from build123d import *

# Parameters (mm, degrees)
EXTRUDE_1_DEPTH     = 5
EXTRUDE_2_DEPTH     = 7
SKETCH_3_R          = 1.5
CUT_EXTRUDE_1_DEPTH = 10
SKETCH_4_R          = 1.6
CUT_EXTRUDE_2_DEPTH = 3.5
SKETCH_5_W          = 8
SKETCH_5_H          = 4
CUT_EXTRUDE_4_DEPTH = 21.784609691
FILLET_1_R          = 5


with BuildPart() as part:
    # 草图1 → 凸台-拉伸1 (new body)
    with BuildSketch(Plane(origin=(0, 0, 0), x_dir=(1, 0, 0), z_dir=(0, 1, 0))):
        with BuildLine():
            ThreePointArc((12, 0), (0, 12), (-12, 0))
            Line((-12, 0), (12, 0))
        make_face()
        with BuildLine():
            ThreePointArc((-12, 0), (-11.422817781, -3.676851089), (-9.746794345, -7))
            Line((-9.746794345, -7), (9.746794345, -7))
            ThreePointArc((9.746794345, -7), (11.422817781, -3.676851089), (12, 0))
            Line((12, 0), (-12, 0))
        make_face()
        with BuildLine():
            Line((-12, 0), (-12, -7))
            Line((-12, -7), (-9.746794345, -7))
            ThreePointArc((-9.746794345, -7), (-11.422817781, -3.676851089), (-12, 0))
        make_face()
        with BuildLine():
            Line((9.746794345, -7), (-9.746794345, -7))
            ThreePointArc((-9.746794345, -7), (0, -12), (9.746794345, -7))
        make_face()
        with BuildLine():
            ThreePointArc((12, 0), (11.422817781, -3.676851089), (9.746794345, -7))
            Line((9.746794345, -7), (12, -7))
            Line((12, -7), (12, 0))
        make_face()
    extrude(amount=EXTRUDE_1_DEPTH)

    # 草图2 → 凸台-拉伸2 (add)
    with BuildSketch(Plane(origin=(0, 5, 0), x_dir=(1, 0, 0), z_dir=(0, 1, 0))):
        with BuildLine():
            Line((-12, 0), (-12, -7))
            Line((-12, -7), (-9.746794345, -7))
            Line((-9.746794345, -7), (9.746794345, -7))
            Line((9.746794345, -7), (12, -7))
            Line((12, -7), (12, 0))
            ThreePointArc((12, 0), (11.827182716, 2.029223745), (11.313708499, 4))
            Line((11.313708499, 4), (-11.313708499, 4))
            ThreePointArc((-11.313708499, 4), (-11.827182716, 2.029223745), (-12, 0))
        make_face()
    extrude(amount=EXTRUDE_2_DEPTH)

    # 草图3 → 切除-拉伸1 (cut)
    with BuildSketch(Plane.XZ):
        with Locations(Location((9, 0, 0), (0, 0, 270))):
            Circle(SKETCH_3_R)
        with Locations(Location((-9, 0, 0), (0, 0, 90))):
            Circle(SKETCH_3_R)
    extrude(amount=-CUT_EXTRUDE_1_DEPTH, mode=Mode.SUBTRACT)

    # 草图4 → 切除-拉伸2 (cut)
    with BuildSketch(Plane.XY.offset(7)):
        with Locations((9, 8)):
            Circle(SKETCH_4_R)
        with Locations(Location((-9, 8, 0), (0, 0, 180))):
            Circle(SKETCH_4_R)
    extrude(amount=-CUT_EXTRUDE_2_DEPTH, mode=Mode.SUBTRACT)

    # 草图5 → 切除-拉伸4 (cut, through all)
    with BuildSketch(Plane(origin=(0, 12, 0), x_dir=(1, 0, 0), z_dir=(0, 1, 0))):
        with Locations((0, 3)):
            Rectangle(SKETCH_5_W, SKETCH_5_H)
    extrude(amount=-CUT_EXTRUDE_4_DEPTH, mode=Mode.SUBTRACT)

    # 圆角1
    # the kernel refuses this fillet: 5 mm, written as the material it adds along each edge
    with BuildSketch(Plane(origin=(-9.746794345, 0, 7), x_dir=(0.6466979741325999, 0, 0.7627461768195178), z_dir=(0, 1, 0))) as fillet_1_piece_1_section:
        with BuildLine():
            CenterArc((2.329688222, -4.983839976), FILLET_1_R, 94.607768722, 45.099127844)
            Line((-1.484042662, -1.750350105), (0, 0))
            ThreePointArc((0, 0), (0.964008919, -0.038784058), (1.928017839, 0))
        make_face()
    fillet_1_piece_1 = extrude(amount=5, mode=Mode.PRIVATE)
    fillet_1_piece_1 = split(fillet_1_piece_1, bisect_by=Plane(origin=(-12, 2.5, 7.309223298), z_dir=(1, 0, 0)), keep=Keep.TOP, mode=Mode.PRIVATE)
    add(fillet_1_piece_1)
    with BuildSketch(Plane(origin=(9.746794345, 0, 7), x_dir=(-0.6466979741326015, 0, 0.7627461768195165), z_dir=(0, 1, 0))) as fillet_1_piece_2_section:
        with BuildLine():
            CenterArc((2.329688222, 4.983839976), FILLET_1_R, 220.293103434, 45.099127844)
            Line((-1.484042662, 1.750350105), (0, 0))
            ThreePointArc((0, 0), (0.964008919, 0.038784058), (1.928017839, 0))
        make_face()
    fillet_1_piece_2 = extrude(amount=5, mode=Mode.PRIVATE)
    fillet_1_piece_2 = split(fillet_1_piece_2, bisect_by=Plane(origin=(12, 2.5, 7.309223298), z_dir=(-1, 0, 0)), keep=Keep.TOP, mode=Mode.PRIVATE)
    add(fillet_1_piece_2)


solid = part.part
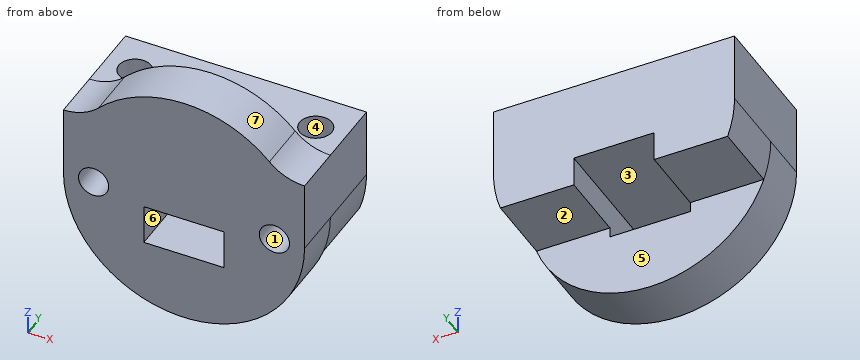
Source: CAD feature listing. Evaluate the final solid. Frame: model axes, mm. Face numbers are marked on the shaded views. A direction names the side the tool comes from. Give positions to 0.01 mm unless a question says otherwise; leave off trailing zeros. Write each loop counter-clockwise with the first axis right and the second up, starting at its lowest first coordinate (ties: lowest second). Pieces come first, ordered by that corner, then holes. Notation, with made-up numbers: M 35.5,75.25 L 68.5,75.25 A32 cw 68.5,103.25 Z; hole C -21,61 d9. An arc over 180 degrees is marked long. Answer as a JSON object with one key per item and string values.
Q1. Cut plane C-C, the plane z = 4.5. Return the cut outline in (x, y).
Geometry check:
{"outline": "M -12,0 L 12,0 L 12,12 L -12,12 Z; hole C -9,8 d3.2; hole C 9,8 d3.2"}
Q2. Contact query for flat-ended pins moving along their axis: P1, Ø2, axis at x = 8, y = 8, coming from the -Z side; P2, Ø1.5, axis at x = 2, z = -7, coming from the +Y side; P3, Ø2.5, axis at x = -9, z = 0, coming from the -Y side; P4, Ø6, axis at x = 0, z = -6, coming from the -Y side. Output: stop coordinate, or through.
Geometry check:
{"P1": "stops at z = -4", "P2": "stops at y = 5", "P3": "stops at y = 10", "P4": "stops at y = 0"}
Q3. Cut plane D-D, the plane y = 3.5. Return the cut outline in (x, z).
Geometry check:
{"outline": "M -12,0 A12 ccw 12,0 L 12,7 A5 cw 8.5,8.47 A12 ccw -8.5,8.47 A5 cw -12,7 Z; hole C -9,0 d3; hole M -4,-5 L 4,-5 L 4,-1 L -4,-1 Z; hole C 9,0 d3"}
Q4. Mould query, pull axis X, two halves, no side actions, for the marked faces 5, 6 and 7. Classes: +X half, -X half, draft (parallel to the pull), parting line (faces both ways), or undercut.
Geometry check:
{"face 5": "draft", "face 6": "undercut", "face 7": "parting line"}
Q5. Access query for the marked faces 1, 2, 3 and 4. Directions: +Z, -Z, +X, -X, +Y, -Y. A direction counts if a zero-diameter tool reaches every point of the face in a straight line with its end or side. Return the directions, or none.
Geometry check:
{"face 1": "-Y", "face 2": "-Z, +X, -X, +Y", "face 3": "+Y, -Y", "face 4": "+Z"}
Q6. Cut plane A-A, the plane x = 0. Return the cut outline in (y, z).
Geometry check:
{"outline": "M 0,-12 L 5,-12 L 5,-5 L 0,-5 Z; M 0,-1 L 12,-1 L 12,7 L 5,7 L 5,12 L 0,12 Z"}
Q7. Cut plane B-B, the plane y = 8. Return the cut outline in (x, z), then the cut area to 3 significant figures.
Geometry check:
{"outline": "M -12,0 A12 ccw -11.31,-4 L -4,-4 L -4,-1 L 4,-1 L 4,-4 L 11.31,-4 A12 ccw 12,0 L 12,7 L 10.6,7 L 10.6,3.5 L 7.4,3.5 L 7.4,7 L -7.4,7 L -7.4,3.5 L -10.6,3.5 L -10.6,7 L -12,7 Z; hole C -9,0 d3; hole C 9,0 d3", "area": "202 mm^2"}
Q8. Ray query, line 1 along X through (y, z) = (8, 0); line 2 along X through (y, z) = (6.75, 0.5); line 3 along Y through (x, z) = (-9.25, 7.5). Return the intervals inside material, ascending.
Geometry check:
{"line 1": "x = -12 to -10.5, -7.5 to 7.5, 10.5 to 12", "line 2": "x = -12 to -10.41, -7.59 to 7.59, 10.41 to 12", "line 3": "y = 0 to 5"}
